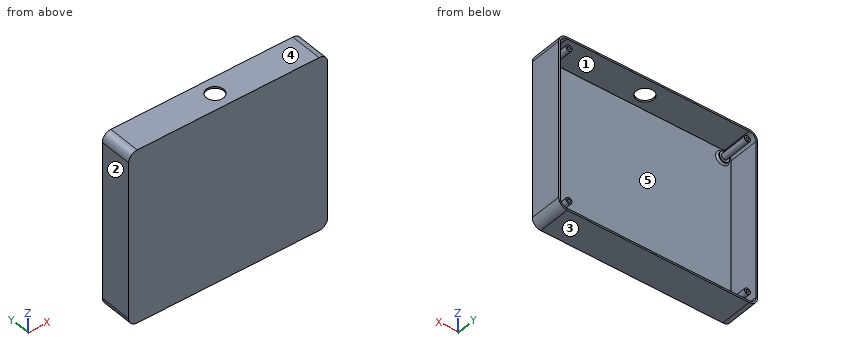
from build123d import *

# Parameters (mm, degrees)
SKETCH1_W            = 231.4
SKETCH1_H            = 201.4
BOSS_EXTRUDE1_DEPTH  = 38
FILLET1_R            = 10
SHELL1_T             = -2
SKETCH2_R            = 10
CUT_EXTRUDE1_DEPTH   = 2
SKETCH3_R            = 6
BOSS_EXTRUDE2_DEPTH  = 3
SKETCH4_R            = 3.5
SKETCH4_R_2          = 1.8
BOSS_EXTRUDE3_DEPTH  = 33
FILLET2_R            = 2
FILLET2_OF_MIRROR1_R = 2


# Read off the part's stored shape, not the designer's step: Mirror2
with BuildPart() as part:
    # Sketch1 → Boss-Extrude1 (new body)
    with BuildSketch(Plane(origin=(0, 0, 0), x_dir=(1, 0, 0), z_dir=(0, 1, 0))):
        Rectangle(SKETCH1_W, SKETCH1_H)
    extrude(amount=BOSS_EXTRUDE1_DEPTH)

    # Fillet1
    fillet1_edges = [part.edges().sort_by_distance(p)[0] for p in [
        (-115.7, 19, -100.7),
        (115.7, 19, -100.7),
        (115.7, 19, 100.7),
        (-115.7, 19, 100.7),
    ]]
    fillet(fillet1_edges, radius=FILLET1_R)

    # Shell1
    shell1_openings = [part.faces().sort_by_distance(p)[0] for p in [
        (0, 38, 0),
    ]]
    offset(amount=SHELL1_T, openings=shell1_openings, kind=Kind.INTERSECTION)

    # Sketch2 → Cut-Extrude1 (cut)
    with BuildSketch(Plane.XY.offset(100.7)):
        with Locations((0, 19)):
            Circle(SKETCH2_R)
    extrude(amount=-CUT_EXTRUDE1_DEPTH, mode=Mode.SUBTRACT)

    # Sketch3 → Boss-Extrude2 (add)
    with BuildSketch(Plane(origin=(0, 2, 0), x_dir=(1, 0, 0), z_dir=(0, 1, 0))):
        with Locations(Location((-103.7, 88.7, 0), (0, 0, 270))):
            Circle(SKETCH3_R)
    boss_extrude2 = extrude(amount=BOSS_EXTRUDE2_DEPTH)

    # Sketch4 → Boss-Extrude3 (add)
    with BuildSketch(Plane(origin=(0, 5, 0), x_dir=(1, 0, 0), z_dir=(0, 1, 0))):
        with Locations(Location((-103.7, 88.7, 0), (0, 0, 270))):
            Circle(SKETCH4_R)
        with Locations(Location((-103.7, 88.7, 0), (0, 0, 270))):
            Circle(SKETCH4_R_2, mode=Mode.SUBTRACT)
    boss_extrude3 = extrude(amount=BOSS_EXTRUDE3_DEPTH)

    # Fillet2
    fillet2_edges = [part.edges().sort_by_distance(p)[0] for p in [
        (-103.7, 2, -94.7),
    ]]
    fillet(fillet2_edges, radius=FILLET2_R)

    # Mirror1: Boss-Extrude2, Boss-Extrude3 across plane
    add(boss_extrude2.mirror(Plane(origin=(0, 0, 0), x_dir=(0, 0, 1), z_dir=(1, 0, 0))))
    add(boss_extrude3.mirror(Plane(origin=(0, 0, 0), x_dir=(0, 0, 1), z_dir=(1, 0, 0))))

    # Fillet2 of Mirror1
    fillet2_of_mirror1_edges = [part.edges().sort_by_distance(p)[0] for p in [
        (103.7, 2, -94.7),
    ]]
    fillet(fillet2_of_mirror1_edges, radius=FILLET2_OF_MIRROR1_R)

    # Mirror2 outline → Mirror2 (revolve)
    with BuildSketch(Plane(origin=(103.7, 0, 88.7), x_dir=(1, 0, 0), z_dir=(0, 0, 1))):
        with BuildLine():
            Line((3.5, 38), (1.8, 38))
            Line((1.8, 38), (1.8, 5))
            Line((1.8, 5), (0, 5))
            Line((0, 5), (0, 2))
            Line((0, 2), (8, 2))
            ThreePointArc((8, 2), (6.585786438, 2.585786438), (6, 4))
            Line((6, 4), (6, 5))
            Line((6, 5), (3.5, 5))
            Line((3.5, 5), (3.5, 38))
        make_face()
    revolve(axis=Axis((103.7, 0, 88.7), (0, 1, 0)))

    # Mirror2 2 outline → Mirror2 2 (revolve)
    with BuildSketch(Plane(origin=(-103.7, 0, 88.7), x_dir=(1, 0, 0), z_dir=(0, 0, 1))):
        with BuildLine():
            Line((3.5, 38), (1.8, 38))
            Line((1.8, 38), (1.8, 5))
            Line((1.8, 5), (0, 5))
            Line((0, 5), (0, 2))
            Line((0, 2), (8, 2))
            ThreePointArc((8, 2), (6.585786438, 2.585786438), (6, 4))
            Line((6, 4), (6, 5))
            Line((6, 5), (3.5, 5))
            Line((3.5, 5), (3.5, 38))
        make_face()
    revolve(axis=Axis((-103.7, 0, 88.7), (0, 1, 0)))


solid = part.part
Design review of the part built by this model. Coordinates are the model's own, in mm. Face numbers are marked on the shaded views. A direction names the side the tool comes from. Give positions to 0.01 mm unless a question says otherwise; leave off trailing zeros. Order: outer loops, then holes, each group sorted by start corner. A loop starts at its lowest first (then second) coordinate and runs counter-clockwise, first axis right, second up. Notation, with made-up numbers: (22.25, 44.5) - (81.25, 44.5) arc R29 cw to (81.25, 73.5) - close; hole circle Ø3 at (30.25, 21.5). An arc over 180 degrees is marked (long way). Use CSV: the item, a comma, the result in double quotes. Start each with the question number.
Q1. Take a section at A-A (y = 19). Count the separate pieces of the cut face and the enclosed holes in it, and give its area (3 significant figures).
Q2. For P1, Ø5, axis at x = 0.5, z = 14.5, coming from the +Y side; P2, Ø1.1, axis at x = 103.5, z = 88, coming from the +Y side, all flat-tipped, find the tip position at first contact; note any pin that passes through.
Q3. Draft analysis for pull direction X (two halves, no side actions). For the marked faces 1, 2 and 3, state which applies: pulls with the +X half, pulls with the -X half, needs draft (parallel to the pull), parting line crosses it, or undercut.
Q4. Take a section at C-C (z = -57.5). State the section outline as (x, y) points.
Q5. Machinability: for the marked faces 4 and 5, which of the approach directions +Z, -Z, +X, -X, +Y, -Y give a long, thin tool a straight path to every point of the face, cutting with its end or side? Answer none if there is none.
Q6. For line 1 (X direction, y = 13, z = -88.7); line 2 (Z direction, x = 103.7, y = 29); line 3 (Z direction, x = -69.5, y = 33), list the stretches that pass through material, from the lowest coordinate up.
Q7. Take a section at D-D (x = -15.5). State the section outline as (y, z) points, and give its area (3 significant figures).
Calculated:
1,separate pieces,"5"
1,enclosed holes,"4"
1,area,"1,760 mm²"
2,P1,"stops at y = 2"
2,P2,"stops at y = 5"
3,face 1,"undercut"
3,face 2,"pulls with the -X half"
3,face 3,"needs draft"
4,outline,"(-115.7, 0) - (115.7, 0) - (115.7, 38) - (113.7, 38) - (113.7, 2) - (-113.7, 2) - (-113.7, 38) - (-115.7, 38) - close"
5,face 4,"+Z, +X, -X, +Y, -Y"
5,face 5,"+Y"
6,line 1,"x = -115.7 to -113.7, -107.2 to -105.5, -101.9 to -100.2, 100.2 to 101.9, 105.5 to 107.2, 113.7 to 115.7"
6,line 2,"z = -100.7 to -98.7, -92.2 to -90.5, -86.9 to -85.2, 85.2 to 86.9, 90.5 to 92.2, 98.7 to 100.7"
6,line 3,"z = -100.7 to -98.7, 98.7 to 100.7"
7,outline,"(0, -100.7) - (38, -100.7) - (38, -98.7) - (2, -98.7) - (2, 98.7) - (38, 98.7) - (38, 100.7) - (0, 100.7) - close"
7,area,"547 mm²"
